CAD build for the part. Positions are in the model's coordinates, mm. A direction names the side the tool comes from. Coordinates: 2 decimals unless noted, no trailing zeros. Loops run counter-clockwise (first coordinate to the right, second up) from the corner with the lowest first, then second, coordinate; pieces in that order, holes last.
1) Saw through at A-A, the plane y = 3. Write the cut outline in (x, z).
2) Saw through at D-D, the plane x = 27. Write the cut outline in (y, z), and give its area (3 significant figures).
3) Saw through at B-B, the plane x = 0. Write the cut outline in (y, z).
4) Which spindle directions (+Z, -Z, +X, -X, +Y, -Y) get a long thin tool onto all of the face, cutting with end or side? Do faces 1 (the flat face through (40, -10, 3)), 2 (the flat face through (40, 10, 3)), 3 (the cylindrical face through (59.22, -14.92, 3.67)), 4 (the flat face through (-18, 13, 5)). Say none if no direction does.
5) Pin check, flat tip, straight feed: pin 1 Ø2 at (x, z) = (50.5, 3.5) entering from +Y. Stop position of the tip, or through.
6) Saw through at C-C, the plane z = 5.25. Give the number of separate pieces and of enclosed holes in the cut face, and give its area (3 significant figures).
7) Wall check: line 1 along X through (y, z) = (-15.45, 3.5); line 2 along X through (y, z) = (11, 5.75); line 3 along X through (y, z) = (6, 3.5). Give the ranges that are in metal, low to high.
8) Two-plate mould, pull along Y, no slides. Class faces 5 (the flat face through (61, 16, 3)), 6 (the flat face through (15, -13, 3)), 7 (the flat face through (-20, 12.2, 5)): +Y half, -Y half, draft (parallel to the pull), parting line (faces both ways), or undercut.
```python
from build123d import *

# Parameters (mm, degrees)
SKETCH_1_R          = 5
EXTRUDE_1_DEPTH     = 7
M2X0_4_1_D          = 1.6
CUT_EXTRUDE_1_DEPTH = 0.8
CUT_EXTRUDE_2_DEPTH = 0.8


with BuildPart() as part:
    # 草图1 → 凸台-拉伸1 (new body)
    with BuildSketch(Plane.XY):
        Polygon((-15, 10), (-15, 16), (-27.5, 16), (-27.5, -16), (-15, -16), (-15, -10), (15, -10), (15, -16), (25, -16), (25, -10), (55, -10), (55, -16), (67.5, -16), (67.5, 16), (55, 16), (55, 10), (25, 10), (25, 16), (15, 16), (15, 10), align=None)
        Circle(SKETCH_1_R, mode=Mode.SUBTRACT)
        with Locations(Location((40, 0, 0), (0, 0, 180))):
            Circle(SKETCH_1_R, mode=Mode.SUBTRACT)
    extrude(amount=EXTRUDE_1_DEPTH)

    # M2x0.4 螺纹孔1 (through all)
    with Locations(Plane(origin=(-20, 16, 3.5), x_dir=(0, 0, 1), z_dir=(0, 1, 0))):
        with Locations((0, 0), (0, 40), (0, 80)):
            Hole(M2X0_4_1_D / 2)

    # 草图4 → 切除-拉伸1 (cut, symmetric)
    with BuildSketch(Plane(origin=(0, 13, 0), x_dir=(1, 0, 0), z_dir=(0, 1, 0))):
        Polygon((-22, -4.654700538), (-22, -7), (-18, -7), (-18, -4.654700538), (-18, -2.345299462), (-20, -1.190598923), (-22, -2.345299462), align=None)
        Polygon((18, -4.654700538), (18, -7), (22, -7), (22, -4.654700538), (22, -2.345299462), (20, -1.190598923), (18, -2.345299462), align=None)
        Polygon((58, -4.654700538), (58, -7), (62, -7), (62, -4.654700538), (62, -2.345299462), (60, -1.190598923), (58, -2.345299462), align=None)
    extrude(amount=CUT_EXTRUDE_1_DEPTH, both=True, mode=Mode.SUBTRACT)

    # 草图5 → 切除-拉伸2 (cut, symmetric)
    with BuildSketch(Plane(origin=(0, -13, 0), x_dir=(-1, 0, 0), z_dir=(0, -1, 0))):
        Polygon((-20, -1.190598923), (-22, -2.345299462), (-22, -4.654700538), (-22, -7), (-18, -7), (-18, -4.654700538), (-18, -2.345299462), align=None)
        Polygon((-60, -1.190598923), (-62, -2.345299462), (-62, -4.654700538), (-62, -7), (-58, -7), (-58, -4.654700538), (-58, -2.345299462), align=None)
        Polygon((20, -1.190598923), (18, -2.345299462), (18, -4.654700538), (18, -7), (22, -7), (22, -4.654700538), (22, -2.345299462), align=None)
    extrude(amount=CUT_EXTRUDE_2_DEPTH, both=True, mode=Mode.SUBTRACT)


solid = part.part
```
Data:
1. outline: (-27.5, 0) - (-4, 0) - (-4, 7) - (-27.5, 7) - close; (4, 0) - (36, 0) - (36, 7) - (4, 7) - close; (44, 0) - (67.5, 0) - (67.5, 7) - (44, 7) - close; hole circle Ø1.6 at (-20, 3.5); hole circle Ø1.6 at (20, 3.5); hole circle Ø1.6 at (60, 3.5)
2. outline: (-10, 0) - (10, 0) - (10, 7) - (-10, 7) - close
2. area: 140 mm2
3. outline: (-10, 0) - (-5, 0) - (-5, 7) - (-10, 7) - close; (5, 0) - (10, 0) - (10, 7) - (5, 7) - close
4. face 1: +Z, -Z, -Y
4. face 2: +Z, -Z, +Y
4. face 3: +Y, -Y
4. face 4: +Z
5. pin 1: stops at y = 10
6. separate pieces: 1
6. enclosed holes: 8
6. area: 2,120 mm2
7. line 1: x = -27.5 to -20.8, -19.2 to -15, 15 to 19.2, 20.8 to 25, 55 to 59.2, 60.8 to 67.5
7. line 2: x = -27.5 to -15, 15 to 25, 55 to 67.5
7. line 3: x = -27.5 to -20.8, -19.2 to 19.2, 20.8 to 59.2, 60.8 to 67.5
8. face 5: +Y half
8. face 6: draft
8. face 7: undercut
